```python
from build123d import *

# Parameters (mm, degrees)
F0_R     = 1.5875
F1_DEPTH = 5.08


with BuildPart() as f1:
    # F0 (on Top) → F1 (new body)
    with BuildSketch(Plane.XY):
        with BuildLine():
            ThreePointArc((27.218649, -26.659991), (35.274924, -14.39756), (38.1, 0))
            ThreePointArc((38.1, 0), (37.997537, 2.792342), (37.690699, 5.569665))
            ThreePointArc((37.690699, 5.569665), (36.235253, 11.773547), (33.766184, 17.648083))
            ThreePointArc((33.766184, 17.648083), (22.394618, 30.823547), (6.35, 37.567107))
            ThreePointArc((6.35, 37.567107), (0, 38.1), (-6.35, 37.567107))
            ThreePointArc((-6.35, 37.567107), (-22.394618, 30.823547), (-33.766184, 17.648083))
            ThreePointArc((-33.766184, 17.648083), (-36.235253, 11.773547), (-37.690699, 5.569665))
            ThreePointArc((-37.690699, 5.569665), (-36.235253, -11.773547), (-27.218649, -26.659991))
            ThreePointArc((-27.218649, -26.659991), (-22.394618, -30.823547), (-16.944133, -34.124864))
            ThreePointArc((-16.944133, -34.124864), (0, -38.1), (16.944133, -34.124864))
            ThreePointArc((16.944133, -34.124864), (22.394618, -30.823547), (27.218649, -26.659991))
        make_face()
        with BuildLine():
            ThreePointArc((33.766184, 17.648083), (36.235253, 11.773547), (37.690699, 5.569665))
            Line((37.690699, 5.569665), (46.749513, 8.513052))
            ThreePointArc((46.749513, 8.513052), (48.59733, 10.091237), (48.787988, 12.513786))
            Line((48.787988, 12.513786), (46.82573, 18.552995))
            ThreePointArc((46.82573, 18.552995), (45.247546, 20.400811), (42.824997, 20.59147))
            Line((42.824997, 20.59147), (33.766184, 17.648083))
        make_face()
        with Locations((45.768384, 11.532657)):
            Circle(F0_R, mode=Mode.SUBTRACT)
        with Locations((43.806126, 17.571866)):
            Circle(F0_R, mode=Mode.SUBTRACT)
        with BuildLine():
            Line((32.817304, -34.365878), (27.218649, -26.659991))
            ThreePointArc((27.218649, -26.659991), (22.394618, -30.823547), (16.944133, -34.124864))
            Line((16.944133, -34.124864), (22.542788, -41.830751))
            ThreePointArc((22.542788, -41.830751), (24.614737, -43.100443), (26.977635, -42.533162))
            Line((26.977635, -42.533162), (32.114893, -38.800725))
            ThreePointArc((32.114893, -38.800725), (33.384585, -36.728776), (32.817304, -34.365878))
        make_face()
        with Locations((25.111417, -39.964533)):
            Circle(F0_R, mode=Mode.SUBTRACT)
        with Locations((30.248675, -36.232096)):
            Circle(F0_R, mode=Mode.SUBTRACT)
        with BuildLine():
            ThreePointArc((-6.35, 37.567107), (0, 38.1), (6.35, 37.567107))
            Line((6.35, 37.567107), (6.35, 47.092107))
            ThreePointArc((6.35, 47.092107), (5.420064, 49.337171), (3.175, 50.267107))
            Line((3.175, 50.267107), (-3.175, 50.267107))
            ThreePointArc((-3.175, 50.267107), (-5.420064, 49.337171), (-6.35, 47.092107))
            Line((-6.35, 47.092107), (-6.35, 37.567107))
        make_face()
        with Locations((-3.175, 47.092107)):
            Circle(F0_R, mode=Mode.SUBTRACT)
        with Locations((3.175, 47.092107)):
            Circle(F0_R, mode=Mode.SUBTRACT)
        with BuildLine():
            Line((-22.542788, -41.830751), (-16.944133, -34.124864))
            ThreePointArc((-16.944133, -34.124864), (-22.394618, -30.823547), (-27.218649, -26.659991))
            Line((-27.218649, -26.659991), (-32.817304, -34.365878))
            ThreePointArc((-32.817304, -34.365878), (-33.384585, -36.728776), (-32.114893, -38.800725))
            Line((-32.114893, -38.800725), (-26.977635, -42.533162))
            ThreePointArc((-26.977635, -42.533162), (-24.614737, -43.100443), (-22.542788, -41.830751))
        make_face()
        with Locations((-25.111417, -39.964533)):
            Circle(F0_R, mode=Mode.SUBTRACT)
        with Locations((-30.248675, -36.232096)):
            Circle(F0_R, mode=Mode.SUBTRACT)
        with BuildLine():
            ThreePointArc((-37.690699, 5.569665), (-36.235253, 11.773547), (-33.766184, 17.648083))
            Line((-33.766184, 17.648083), (-42.824997, 20.59147))
            ThreePointArc((-42.824997, 20.59147), (-45.247546, 20.400811), (-46.82573, 18.552995))
            Line((-46.82573, 18.552995), (-48.787988, 12.513786))
            ThreePointArc((-48.787988, 12.513786), (-48.59733, 10.091237), (-46.749513, 8.513052))
            Line((-46.749513, 8.513052), (-37.690699, 5.569665))
        make_face()
        with Locations((-45.768384, 11.532657)):
            Circle(F0_R, mode=Mode.SUBTRACT)
        with Locations((-43.806126, 17.571866)):
            Circle(F0_R, mode=Mode.SUBTRACT)
    extrude(amount=F1_DEPTH)


solid = f1.part
```
Input: part model. Units: mm. Frame: model coordinates. A direction names the side the tool comes from. Give positions to 0.01 mm unless a question says otherwise; leave off trailing zeros. Order: outer loops, then holes, each group sorted by start corner. A loop starts at its lowest first (then second) coordinate and runs counter-clockwise, first axis right, second up. Notation, with made-up numbers: (-29, 36) -> (30, 36) arc R26 cw to (30, 55) -> close; hole circle Ø9 at (-14.75, -24.5). An arc over 180 degrees is marked (long way). Write each question's results on one line, items separated by ' | '. Start each with the question number.
Item 1: Line query: line 1 (Y direction, x = 44.5, z = 4.1); line 2 (Y direction, x = -31, z = 1.4); line 3 (X direction, y = 12, z = 3.7). Output: solid intervals per line, ascending.
Item 2: Cut plane A-A on y = 41. Return the cut outline in (x, z), then the cut area to 3 significant figures.
Item 3: Set-up query: faces 5 (the cylindrical face through (5.445, 49.312, 2.504)), 6 (the flat face through (-38.23, 19.1, 2.5)), 7 (the flat face through (-19.78, -38.03, 2.5)). Return all of +Z, -Z, +X, -X, +Y, -Y with unobstructed straight access to the full face (end or side cutting, diameter ignored); none if empty.
Item 4: Contact query for flat-ended pins moving along their axis: P1, Ø2.5, axis at x = 45.77, y = 11.53, coming from the +Z side; P2, Ø1.5, axis at y = 42, z = 2.5, coming from the +X side; P3, Ø5, axis at x = -3.18, y = 47.09, coming from the -Z side; P4, Ø2.5, axis at y = 42, z = 3.5, coming from the -X side. Output: stop coordinate, or through.
Item 5: Cut plane C-C on x = 7.5. Return the cut outline in (y, z), then the cut area to 3 significant figures.
Item 6: Cut plane B-B on z = 2. Give the number of separate pieces and of enclosed holes in the cut face, then the cut area to 3 significant figures.
Item 7: Mould query, pull axis Y, two halves, no side actions, for faces 1 (the flat face through (38.36, 19.14, 2.5)), 2 (the flat face through (-1, 4, 0)), 3 (the cylindrical face through (-47.03, 10.57, 2.5)), 4 (the cylindrical face through (2.005, 48.165, 2.504)). Classes: pulls with the +Y half, pulls with the -Y half, needs draft (parallel to the pull), parting line crosses it, or undercut.
Established:
1) line 1: 7.78 to 10.58, 12.49 to 16.14, 19 to 20.67 | line 2: -39.61 to -37.63, -34.83 to -31.86, -22.15 to 22.15 | line 3: -48.91 to -47.29, -44.25 to 44.25, 47.29 to 48.91
2) outline: (-6.35, 0) -> (6.35, 0) -> (6.35, 5.08) -> (-6.35, 5.08) -> close | area: 64.5 mm^2
3) face 5: +Z, -Z, +X, +Y | face 6: +Z, -Z, +Y | face 7: +Z, -Z, -Y
4) P1: through | P2: x = 6.35 | P3: z = 0 | P4: x = -6.35
5) outline: (-37.35, 0) -> (37.35, 0) -> (37.35, 5.08) -> (-37.35, 5.08) -> close | area: 380 mm^2
6) separate pieces: 1 | enclosed holes: 10 | area: 5,240 mm^2
7) face 1: pulls with the +Y half | face 2: needs draft | face 3: undercut | face 4: undercut
